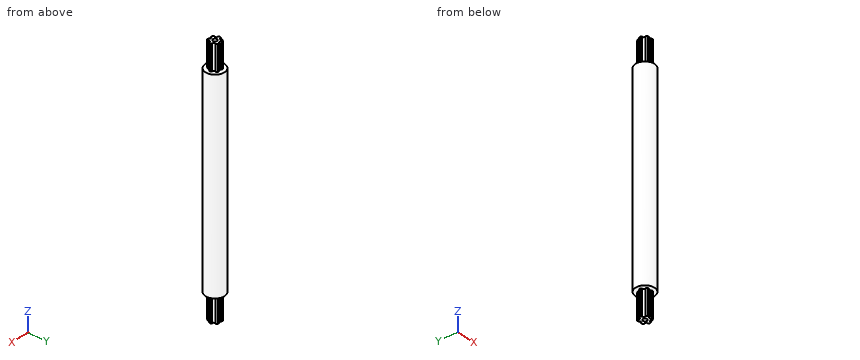
from build123d import *

# Parameters (mm, degrees)
SKETCH1_R           = 2.54
BOSS_EXTRUDE1_DEPTH = 304.8
SKETCH2_R           = 11.43
BOSS_EXTRUDE2_DEPTH = 121.92


with BuildPart() as part:
    # Sketch1 → Boss-Extrude1 (new body)
    with BuildSketch(Plane.XY):
        with BuildLine():
            Line((7.493, 0), (6.396528537, 1.899144284))
            ThreePointArc((6.396528537, 1.899144284), (4.274330108, 2.467785639), (4.842971463, 4.589984067))
            Line((4.842971463, 4.589984067), (3.7465, 6.489128351))
            Line((3.7465, 6.489128351), (1.553557073, 6.489128351))
            ThreePointArc((1.553557073, 6.489128351), (0, 4.935571277), (-1.553557073, 6.489128351))
            Line((-1.553557073, 6.489128351), (-3.7465, 6.489128351))
            Line((-3.7465, 6.489128351), (-4.842971463, 4.589984067))
            ThreePointArc((-4.842971463, 4.589984067), (-4.274330108, 2.467785639), (-6.396528537, 1.899144284))
            Line((-6.396528537, 1.899144284), (-7.493, 0))
            Line((-7.493, 0), (-6.396528537, -1.899144284))
            ThreePointArc((-6.396528537, -1.899144284), (-4.274330108, -2.467785639), (-4.842971463, -4.589984067))
            Line((-4.842971463, -4.589984067), (-3.7465, -6.489128351))
            Line((-3.7465, -6.489128351), (-1.553557073, -6.489128351))
            ThreePointArc((-1.553557073, -6.489128351), (0, -4.935571277), (1.553557073, -6.489128351))
            Line((1.553557073, -6.489128351), (3.7465, -6.489128351))
            Line((3.7465, -6.489128351), (4.842971463, -4.589984067))
            ThreePointArc((4.842971463, -4.589984067), (4.274330108, -2.467785639), (6.396528537, -1.899144284))
            Line((6.396528537, -1.899144284), (7.493, 0))
        make_face()
        with Locations(Location((0, 0, 0), (0, 0, 180))):
            Circle(SKETCH1_R, mode=Mode.SUBTRACT)
    extrude(amount=BOSS_EXTRUDE1_DEPTH)

    # Sketch2 → Boss-Extrude2 (add, symmetric)
    with BuildSketch(Plane(origin=(0, 0, 152.4), x_dir=(-1, 0, 0), z_dir=(0, 0, -1))):
        with Locations(Location((0, 0, 0), (0, 0, 180))):
            Circle(SKETCH2_R)
    extrude(amount=BOSS_EXTRUDE2_DEPTH, both=True)


solid = part.part
Verification items for the finished model (mm, model axes). Give positions to 0.01 mm unless a question says otherwise; leave off trailing zeros. Write each loop counter-clockwise with the first axis right and the second up, starting at its lowest first coordinate (ties: lowest second). Pieces come first, ordered by that corner, then holes. Notation, with made-up numbers: (63, 46.5) -> (118, 46.5) arc R32 ccw to (118, 74.5) -> close; hole circle Ø11 at (43.5, 42). An arc over 180 degrees is marked (long way). Use CSV: the item, a comma, the result in double quotes.
(1) Material ranges on L1, parallel to Y at x = 0, z = 297.5; L2, parallel to Y at x = 4.5, z = 20; L3, parallel to Z at x = -1.75, y = -7, recorded low to high.
Derived:
L1,"y = -4.94 to -2.54, 2.54 to 4.94"
L2,"y = -5.18 to -4.32, -2.17 to 2.17, 4.32 to 5.18"
L3,"z = 30.48 to 274.32"
(2) Sectioned sample at A-A (z = 173.5). Record the cut outline in (x, y), plus the area to 3 significant figures.
Derived:
outline,"circle Ø22.86 at (0, 0)"
area,"410 mm^2"
(3) Go/stop test with flat-tipped pins: pin 1 (1.5 mm diameter, centred on x = -6, y = -5.5, fed in from +Z); pin 2 (10 mm diameter, centred on x = -7.5, z = 124, fed in from -Y); pin 3 (2.5 mm diameter, centred on x = -3, z = 292.5, fed in from +Y). Record where each tip stops, or that it passes through.
Derived:
pin 1,"stops at z = 274.32"
pin 2,"stops at y = -11.15"
pin 3,"stops at y = 6.49"
